The model under review builds one solid part; all positions refer to its coordinate system, in mm. Face numbers are marked on the shaded views. A direction names the side the tool comes from. Coordinates: 2 decimals unless noted, no trailing zeros. Loops run counter-clockwise (first coordinate to the right, second up) from the corner with the lowest first, then second, coordinate; pieces in that order, holes last. Notation, with made-up numbers: M -19.5,71.5 L 15.5,71.5 A18 ccw 15.5,96.5 Z; hole C 13.5,15.25 d3. An arc over 180 degrees is marked long. One line per item, written item: value.
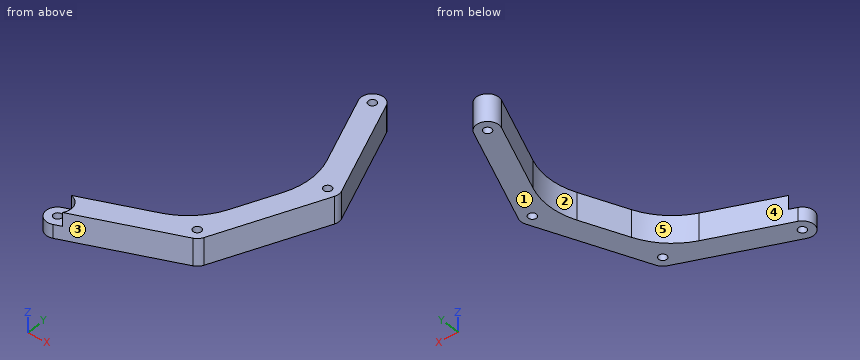
```python
from build123d import *

# Parameters (mm, degrees)
BOSS_EXTRUDE1_DEPTH     = 5
SKETCH2_R               = 2.5
CUT_EXTRUDE1_DEPTH      = 2.5
CUT_EXTRUDE2_DEPTH      = 42.668225696
CUT_EXTRUDE2_DEPTH_BACK = 42.668225696
SKETCH3_R               = 0.75
CUT_EXTRUDE3_DEPTH      = 42.892613104
CUT_EXTRUDE3_DEPTH_BACK = 42.892613104
SKETCH4_R               = 0.75


with BuildPart() as part:
    # Sketch1 → Boss-Extrude1 (new body)
    with BuildSketch(Plane.XY):
        with BuildLine():
            Line((21.247555139, 20.121649117), (29.252444861, 0.796135783))
            ThreePointArc((29.252444861, 0.796135783), (29.410806115, 0), (29.252444861, -0.796135783))
            Line((29.252444861, -0.796135783), (21.247555139, -20.121649117))
            ThreePointArc((21.247555139, -20.121649117), (20.796580444, -20.796580444), (20.121649117, -21.247555139))
            Line((20.121649117, -21.247555139), (0.796135783, -29.252444861))
            ThreePointArc((0.796135783, -29.252444861), (-1.922041804, -28.12653884), (-0.796135783, -25.408361253))
            Line((-0.796135783, -25.408361253), (12.873162178, -19.74635265))
            ThreePointArc((12.873162178, -19.74635265), (16.993338708, -16.993338708), (19.74635265, -12.873162178))
            Line((19.74635265, -12.873162178), (23.065480134, -4.860079591))
            ThreePointArc((23.065480134, -4.860079591), (24.032210071, 0), (23.065480134, 4.860079591))
            Line((23.065480134, 4.860079591), (17.40347153, 18.529377552))
            ThreePointArc((17.40347153, 18.529377552), (18.529377552, 21.247555139), (21.247555139, 20.121649117))
        make_face()
    extrude(amount=BOSS_EXTRUDE1_DEPTH)

    # Sketch2 → Cut-Extrude1 (cut)
    with BuildSketch(Plane.XY.offset(5)):
        with Locations((0, -27.330403057)):
            Circle(SKETCH2_R)
    extrude(amount=-CUT_EXTRUDE1_DEPTH, mode=Mode.SUBTRACT)

    # Sketch3 → Cut-Extrude2 (cut, two sides: drawn at the far end of the back side and taken through both)
    with BuildSketch(Plane.XY.offset(2.5).offset(-CUT_EXTRUDE2_DEPTH_BACK)):
        with Locations((0, -27.330403057)):
            Circle(SKETCH3_R)
    extrude(amount=CUT_EXTRUDE2_DEPTH + CUT_EXTRUDE2_DEPTH_BACK, mode=Mode.SUBTRACT)

    # Sketch4 → Cut-Extrude3 (cut, two sides: drawn at the far end of the back side and taken through both)
    with BuildSketch(Plane(origin=(0, 0, 0), x_dir=(-1, 0, 0), z_dir=(0, 0, -1)).offset(-CUT_EXTRUDE3_DEPTH_BACK)):
        with Locations((-19.325513334, 19.325513334)):
            Circle(SKETCH4_R)
        with Locations((-27.330403057, 0)):
            Circle(SKETCH4_R)
        with Locations((-19.325513334, -19.325513334)):
            Circle(SKETCH4_R)
    extrude(amount=CUT_EXTRUDE3_DEPTH + CUT_EXTRUDE3_DEPTH_BACK, mode=Mode.SUBTRACT)


solid = part.part
```
(1) Tool access review of the marked faces 4 and 5: name each direction out of +Z, -Z, +X, -X, +Y, -Y from which nothing blocks a thin tool from reaching the whole face with its end or side.
Checks:
face 4: +Z, -Z, -X, +Y
face 5: +Z, -Z, -X
(2) Add section B-B on x = 0. State the section outline as (y, z) points, then the cut area to 3 significant figures.
Checks:
outline: M -29.41,0 L -28.08,0 L -28.08,2.5 L -29.41,2.5 Z; M -26.58,0 L -25.08,0 L -25.08,2.5 L -26.58,2.5 Z
area: 7.08 mm^2
(3) Add section C-C on z = 4.35. State the section outline as (x, y) points.
Checks:
outline: M 0.48,-24.88 A2.5 cw 2.08,-28.72 L 20.12,-21.25 A2.08 ccw 21.25,-20.12 L 29.25,-0.8 A2.08 ccw 29.25,0.8 L 21.25,20.12 A2.08 ccw 17.4,18.53 L 23.07,4.86 A12.7 cw 23.07,-4.86 L 19.75,-12.87 A12.7 cw 12.87,-19.75 Z; hole C 19.33,-19.33 d1.5; hole C 19.33,19.33 d1.5; hole C 27.33,0 d1.5
(4) Insertion check: pin 1 Ø1.4 at (x, y) = (19.33, 19.33) entering from +Z; pin 2 Ø3 at (y, z) = (16, 1) entering from +X; pin 3 Ø1.5 at (y, z) = (13, 2.5) entering from +X; pin 4 Ø1 at (y, z) = (12.5, 1.5) entering from +X. Each pin has a flat end and moves straight along its axis. Give the tip position at first contact, or say it passes through.
Checks:
pin 1: through
pin 2: x = 23.58
pin 3: x = 24.51
pin 4: x = 24.61
(5) Add section A-A on y = 0. State the section outline as (x, z) points, then the cut area to 3 significant figures.
Checks:
outline: M 24.03,0 L 26.58,0 L 26.58,5 L 24.03,5 Z; M 28.08,0 L 29.41,0 L 29.41,5 L 28.08,5 Z
area: 19.4 mm^2
(6) Add section D-D on z = 1.3. State the section outline as (x, y) points.
Checks:
outline: M -0.8,-25.41 A2.08 ccw 0.8,-29.25 L 20.12,-21.25 A2.08 ccw 21.25,-20.12 L 29.25,-0.8 A2.08 ccw 29.25,0.8 L 21.25,20.12 A2.08 ccw 17.4,18.53 L 23.07,4.86 A12.7 cw 23.07,-4.86 L 19.75,-12.87 A12.7 cw 12.87,-19.75 Z; hole C 0,-27.33 d1.5; hole C 19.33,-19.33 d1.5; hole C 19.33,19.33 d1.5; hole C 27.33,0 d1.5
(7) To check wall thickness, follow L1, parallel to X at y = 0, z = 3.65; L2, parallel to Y at x = 0.5, z = 0.7; L3, parallel to Y at x = 20, z = 2.25. State the ranges of each line that lie inside material, in increasing order. Write a range as [from, to].
Checks:
L1: [24.03, 26.58], [28.08, 29.41]
L2: [-29.35, -27.89], [-26.77, -24.87]
L3: [-21.3, -19.65], [-19, -12.26], [12.26, 19], [19.65, 21.29]
(8) Draft analysis for pull direction Y (two halves, no side actions). For the marked faces 1, 2 and 3, state which applies: pulls with the +Y half, pulls with the -Y half, needs draft (parallel to the pull), parting line crosses it, or undercut.
Checks:
face 1: needs draft
face 2: undercut
face 3: pulls with the -Y half
